from build123d import *

# Parameters (mm, degrees)
SKETCH1_W            = 72
SKETCH1_H            = 28
SKETCH1_R            = 1.25
SKETCH1_R_2          = 0.5
BOSS_EXTRUDE1_DEPTH  = 1.6
SKETCH2_W            = 35.56
SKETCH2_H            = 17.78
BOSS_EXTRUDE2_DEPTH  = 3.86
BOSS_EXTRUDE3_DEPTH  = 3
SKETCH4_W            = 3
SKETCH4_H            = 5
BOSS_EXTRUDE4_DEPTH  = 1.8
BOSS_EXTRUDE5_DEPTH  = 0.7
BOSS_EXTRUDE6_DEPTH  = 4.09
SKETCH7_W            = 15.7
SKETCH7_H            = 6.2
BOSS_EXTRUDE7_DEPTH  = 8
SKETCH8_W            = 30
SKETCH8_H            = 13
BOSS_EXTRUDE8_DEPTH  = 1.5
SKETCH9_W            = 6
SKETCH9_H            = 20.007270078
BOSS_EXTRUDE9_DEPTH  = 8
SKETCH10_W           = 36.5
SKETCH10_H           = 29
BOSS_EXTRUDE10_DEPTH = 6
SKETCH12_W           = 7.01
SKETCH12_H           = 4.5
BOSS_EXTRUDE11_DEPTH = 5.79
BOSS_EXTRUDE12_DEPTH = 1.27


with BuildPart() as part:
    # Sketch1 → Boss-Extrude1 (new body)
    with BuildSketch(Plane(origin=(0, 0, 0), x_dir=(1, 0, 0), z_dir=(0, 1, 0))):
        Rectangle(SKETCH1_W, SKETCH1_H)
        with Locations(Location((-33, -11, 0), (0, 0, 270))):
            Circle(SKETCH1_R, mode=Mode.SUBTRACT)
        with Locations(Location((28, -11, 0), (0, 0, 270))):
            Circle(SKETCH1_R, mode=Mode.SUBTRACT)
        with Locations(Location((-30.96, 1.27, 0), (0, 0, 270))):
            Circle(SKETCH1_R_2, mode=Mode.SUBTRACT)
        with Locations(Location((28, 11, 0), (0, 0, 90))):
            Circle(SKETCH1_R, mode=Mode.SUBTRACT)
        with Locations(Location((-30.96, -1.27, 0), (0, 0, 90))):
            Circle(SKETCH1_R_2, mode=Mode.SUBTRACT)
    extrude(amount=BOSS_EXTRUDE1_DEPTH)

    # Sketch2 → Boss-Extrude2 (add)
    with BuildSketch(Plane(origin=(0, 1.6, 0), x_dir=(1, 0, 0), z_dir=(0, 1, 0))):
        with Locations((-17.22, 0.01)):
            Rectangle(SKETCH2_W, SKETCH2_H)
    extrude(amount=BOSS_EXTRUDE2_DEPTH)

    # Sketch3 → Boss-Extrude3 (add)
    with BuildSketch(Plane(origin=(0, 5.46, 0), x_dir=(1, 0, 0), z_dir=(0, 1, 0))):
        Polygon((-35, 3.76), (-30, 3.76), (-30, -3.74), (-35, -3.74), (-35.7, -4.02), (-35.7, 4.04), align=None)
    extrude(amount=BOSS_EXTRUDE3_DEPTH)

    # Sketch4 → Boss-Extrude4 (add)
    with BuildSketch(Plane(origin=(0, 5.46, 0), x_dir=(1, 0, 0), z_dir=(0, 1, 0))):
        with Locations((-3.76, 0.01)):
            Rectangle(SKETCH4_W, SKETCH4_H)
    extrude(amount=BOSS_EXTRUDE4_DEPTH)

    # Sketch5 → Boss-Extrude5 (add)
    with BuildSketch(Plane(origin=(0, 7.26, 0), x_dir=(1, 0, 0), z_dir=(0, 1, 0))):
        with BuildLine():
            Line((-2.66, 1.11), (-2.66, -1.09))
            ThreePointArc((-2.66, -1.09), (-3.76, -2.19), (-4.86, -1.09))
            Line((-4.86, -1.09), (-4.86, 1.11))
            ThreePointArc((-4.86, 1.11), (-3.76, 2.21), (-2.66, 1.11))
        make_face()
    extrude(amount=BOSS_EXTRUDE5_DEPTH)

    # Sketch6 → Boss-Extrude6 (add)
    with BuildSketch(Plane(origin=(0, 1.6, 0), x_dir=(1, 0, 0), z_dir=(0, 1, 0))):
        with BuildLine():
            Line((4.315, 10.27), (25.905, 10.27))
            ThreePointArc((25.905, 10.27), (27.701051224, 9.526051224), (28.445, 7.73))
            Line((28.445, 7.73), (28.445, -7.51))
            ThreePointArc((28.445, -7.51), (27.701051224, -9.306051224), (25.905, -10.05))
            Line((25.905, -10.05), (4.315, -10.05))
            ThreePointArc((4.315, -10.05), (2.518948776, -9.306051224), (1.775, -7.51))
            Line((1.775, -7.51), (1.775, 7.73))
            ThreePointArc((1.775, 7.73), (2.518948776, 9.526051224), (4.315, 10.27))
        make_face()
    extrude(amount=BOSS_EXTRUDE6_DEPTH)

    # Sketch7 → Boss-Extrude7 (add)
    with BuildSketch(Plane(origin=(0, 1.6, 0), x_dir=(1, 0, 0), z_dir=(0, 1, 0))):
        with Locations((-18.8, 13)):
            Rectangle(SKETCH7_W, SKETCH7_H)
        with Locations((-3.04, 13)):
            Rectangle(SKETCH7_W, SKETCH7_H)
        with Locations((-3.04, -12.98)):
            Rectangle(SKETCH7_W, SKETCH7_H)
        with Locations((-18.8, -12.98)):
            Rectangle(SKETCH7_W, SKETCH7_H)
    extrude(amount=BOSS_EXTRUDE7_DEPTH)

    # Sketch8 → Boss-Extrude8 (add)
    with BuildSketch(Plane(origin=(0, 0, 0), x_dir=(-1, 0, 0), z_dir=(0, -1, 0))):
        with Locations((-17.55, 0.22970015)):
            Rectangle(SKETCH8_W, SKETCH8_H)
    extrude(amount=BOSS_EXTRUDE8_DEPTH)

    # Sketch9 → Boss-Extrude9 (add)
    with BuildSketch(Plane(origin=(0, 1.6, 0), x_dir=(1, 0, 0), z_dir=(0, 1, 0))):
        with Locations((34, 0)):
            Rectangle(SKETCH9_W, SKETCH9_H)
    extrude(amount=BOSS_EXTRUDE9_DEPTH)

    # Sketch10 → Boss-Extrude10 (add)
    with BuildSketch(Plane(origin=(0, 0, 0), x_dir=(-1, 0, 0), z_dir=(0, -1, 0))):
        with Locations((7.281732971, 0.01)):
            Rectangle(SKETCH10_W, SKETCH10_H)
    extrude(amount=BOSS_EXTRUDE10_DEPTH)

    # Sketch12 → Boss-Extrude11 (add)
    with BuildSketch(Plane(origin=(0, 1.6, 0), x_dir=(1, 0, 0), z_dir=(0, 1, 0))):
        with Locations((-31.75, 11.5)):
            Rectangle(SKETCH12_W, SKETCH12_H)
    extrude(amount=BOSS_EXTRUDE11_DEPTH)

    # Sketch13 → Boss-Extrude12 (add)
    with BuildSketch(Plane(origin=(0, 7.39, 0), x_dir=(1, 0, 0), z_dir=(0, 1, 0))):
        with BuildLine():
            Line((-31.88, 13.53), (-31.62, 13.53))
            ThreePointArc((-31.62, 13.53), (-29.59, 11.5), (-31.62, 9.47))
            Line((-31.62, 9.47), (-31.88, 9.47))
            ThreePointArc((-31.88, 9.47), (-33.91, 11.5), (-31.88, 13.53))
        make_face()
    extrude(amount=BOSS_EXTRUDE12_DEPTH)


solid = part.part
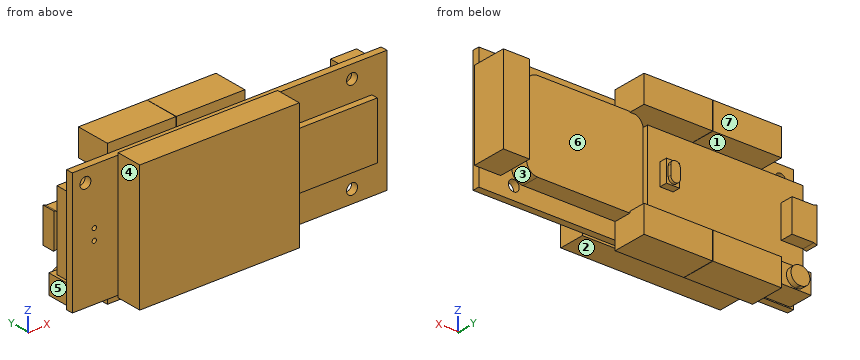
Work out the finished part from the listing and answer in its coordinate system (mm). Face numbers are marked on the shaded views. A direction names the side the tool comes from. Round coordinates to 2 decimals unless told otherwise and drop trailing zeros. Write each loop counter-clockwise with the first axis right and the second up, starting at its lowest first coordinate (ties: lowest second). Pieces come first, ordered by that corner, then holes.
1) Straight lines are drawn through the part: line 1 (X direction, y = 1.15, z = 11); line 2 (Z direction, x = -9.5, y = 3.5); line 3 (Z direction, x = -10.5, y = 7). For each, find the intervals that lie inside material, in ascending order.
2) A cutting plane is placed at A-A (z = 11). Give the vertices of the cut face in (x, y).
3) Given pin 1 Ø6.5 at (x, y) = (35, 6.5) entering from -Z; pin 2 Ø1 at (x, y) = (3, -3) entering from -Z; pin 3 Ø9 at (x, z) = (-9.5, -4.5) entering from +Y, each flat-ended and moving along its own axis, determine where each tip first touches the part or whether it passes through.
4) The mould has two halves that part along X. Classify the marked faces 5, 6 and 7: pulls with the +X half, pulls with the -X half, needs draft (parallel to the pull), parting line crosses it, or undercut.
5) A tool of negligible diameter and unlimited length cuts with its end or side. For the marked faces 1, 2, 3 and 4, from which of +Z, -Z, +X, -X, +Y, -Y can it reach the whole face along a straight path? Write none if from no direction.
6) A cutting plane is placed at B-B (y = 6.5). Give the number of separate pieces and of enclosed holes in the cut face, plus the area to 3 significant figures.
7) A cutting plane is placed at D-D (z = -11). Give the vertices of the cut face in (x, y) (3 decimals).
8) A cutting plane is placed at C-C (x = -3.76). Give the vertices of the cut face in (y, z).
Completed:
1. line 1: x = -36 to -34.25, -31.75 to 26.75, 29.25 to 36
1. line 2: z = -16.1 to -9.9, -8.9 to 8.88, 9.88 to 16.08
1. line 3: z = -16.1 to -9.9, 9.88 to 16.08
2. outline: (-36, 0) - (-34.25, 0) - (-34.25, 1.6) - (-36, 1.6) - close; (-31.75, 0) - (-25.53, 0) - (-25.53, -6) - (10.97, -6) - (10.97, 0) - (26.75, 0) - (26.75, 1.6) - (4.81, 1.6) - (4.81, 9.6) - (-10.89, 9.6) - (-10.89, 1.6) - (-10.95, 1.6) - (-10.95, 9.6) - (-26.65, 9.6) - (-26.65, 1.6) - (-31.75, 1.6) - close; (29.25, 0) - (36, 0) - (36, 1.6) - (29.25, 1.6) - close
3. pin 1: stops at z = -10
3. pin 2: stops at z = -14.51
3. pin 3: stops at y = 5.46
4. face 5: pulls with the -X half
4. face 6: undercut
4. face 7: needs draft
5. face 1: -X, +Y
5. face 2: -Z, +X, -X, -Y
5. face 3: -Z, +Y
5. face 4: +Z, -Z, -X, -Y
6. separate pieces: 8
6. enclosed holes: 0
6. area: 599 mm2
7. outline: (-36, 0) - (-25.532, 0) - (-25.532, -6) - (10.968, -6) - (10.968, 0) - (26.75, 0) - (26.75, 1.6) - (4.81, 1.6) - (4.81, 9.6) - (-10.89, 9.6) - (-10.89, 1.6) - (-10.95, 1.6) - (-10.95, 9.6) - (-26.65, 9.6) - (-26.65, 1.6) - (-28.245, 1.6) - (-28.245, 7.39) - (-29.653, 7.39) - (-29.653, 8.66) - (-33.847, 8.66) - (-33.847, 7.39) - (-35.255, 7.39) - (-35.255, 1.6) - (-36, 1.6) - close; (29.25, 0) - (36, 0) - (36, 1.6) - (29.25, 1.6) - close
8. outline: (-6, -14.51) - (0, -14.51) - (0, -14) - (1.6, -14) - (1.6, -16.1) - (9.6, -16.1) - (9.6, -9.9) - (1.6, -9.9) - (1.6, -8.9) - (5.46, -8.9) - (5.46, -2.51) - (7.26, -2.51) - (7.26, -2.21) - (7.96, -2.21) - (7.96, 2.19) - (7.26, 2.19) - (7.26, 2.49) - (5.46, 2.49) - (5.46, 8.88) - (1.6, 8.88) - (1.6, 9.88) - (9.6, 9.88) - (9.6, 16.08) - (1.6, 16.08) - (1.6, 14) - (0, 14) - (0, 14.49) - (-6, 14.49) - close
